Geometry check sheet. Reference: the model listing, model coordinates, mm. A direction names the side the tool comes from. Round coordinates to 2 decimals unless told otherwise and drop trailing zeros. Write each loop counter-clockwise with the first axis right and the second up, starting at its lowest first coordinate (ties: lowest second). Pieces come first, ordered by that corner, then holes. Notation, with made-up numbers: M 19.5,-33 L 27.5,-33 A18 ccw 27.5,-22 Z; hole C -7.5,8.25 d11. An arc over 180 degrees is marked long. Put each result on its own line as item: value. Start each with the question number.
(1) Tool access check on faces 4 (the flat face through (-40, 0, 13)), 5 (the flat face through (15, -15, 37)), 6 (the flat face through (40, 0, 13)). Record the directions out of +Z, -Z, +X, -X, +Y, -Y that give a thin tool (end or side, any length) a straight path to the whole face; none if there is none.
(2) Mould release check, pull along Y, two halves, no side actions. Record for faces 1 (the flat face through (50, -13, 13)), 2 (the flat face through (15, 15, 37)), 3 (the flat face through (-60, 21, 12)): pulls with the +Y half, pulls with the -Y half, needs draft (parallel to the pull), parting line crosses it, or undercut.
(3) Section check B-B on x = -50.5. Record the cut outline in (y, z), then the cut area to 3 significant figures.
(4) Section check D-D on x = 27. Record the cut outline in (y, z).
(5) Gauge pin test, flat ends, axial feed: pin 1 (10 mm diameter, centred on x = -30, y = -21.5, fed in from +Z); pin 2 (7.5 mm diameter, centred on y = 2, z = 14.5, fed in from +X); pin 3 (5 mm diameter, centred on x = -20.5, z = 28.5, fed in from -Y). Record the tip position at first contact, or that the pin passes through.
(6) Material ranges on probe 1 along Y at (x, z) = (-44.5, 9.5); probe 2 along Z at (x, y) = (-30.5, -11.5); probe 3 along X at (y, z) = (9, 15), recorded low to high.
(7) Section check A-A on z = 32.5. Record the cut outline in (x, y).
(8) Section check C-C on y = 22.5. Record the cut outline in (x, z).
from build123d import *

# Parameters (mm, degrees)
F0_W      = 120
F0_H      = 60
F1_DEPTH  = 25
F2_W      = 20
F2_H      = 26
F3_DEPTH  = 25.001
F4_W      = 20
F4_H      = 26
F5_DEPTH  = 25.001
F7_DEPTH  = 25
F8_DEPTH  = 35.001
F10_DEPTH = 25


with BuildPart() as f1:
    # F0 (on Top) → F1 (new body)
    with BuildSketch(Plane.XY):
        Rectangle(F0_W, F0_H)
    extrude(amount=F1_DEPTH)

    # F2 (on face) → F3 (cut, through all)
    with BuildSketch(Plane.XY.offset(25)):
        with Locations((50, 0)):
            Rectangle(F2_W, F2_H)
    extrude(amount=-F3_DEPTH, mode=Mode.SUBTRACT)

    # F4 (on face) → F5 (cut, through all)
    with BuildSketch(Plane.XY.offset(25)):
        with Locations((-50, 0)):
            Rectangle(F4_W, F4_H)
    extrude(amount=-F5_DEPTH, mode=Mode.SUBTRACT)

    # F6 (on face) → F7 (cut)
    with BuildSketch(Plane.XZ.offset(30)):
        with BuildLine():
            Line((-18, 0), (18, 0))
            ThreePointArc((18, 0), (0, 18), (-18, 0))
        make_face()
    extrude(amount=-F7_DEPTH, mode=Mode.SUBTRACT)

    # F8 (cut, through all): a face of the model
    f8_faces = [f1.faces().sort_by_distance(p)[0] for p in [
        (0, -5, 7.6394372684),
    ]]
    extrude(f8_faces, amount=-F8_DEPTH, mode=Mode.SUBTRACT)

    # F9 (on face) → F10 (join)
    with BuildSketch(Plane.XY.offset(25)):
        with BuildLine():
            ThreePointArc((0, 11), (7.7781745931, 7.7781745931), (11, 0))
            Line((11, 0), (30, 0))
            Line((30, 0), (0, 30))
            Line((0, 30), (0, 11))
        make_face()
        with BuildLine():
            ThreePointArc((-11, 0), (-7.7781745931, 7.7781745931), (0, 11))
            Line((0, 11), (0, 30))
            Line((0, 30), (-30, 0))
            Line((-30, 0), (-11, 0))
        make_face()
        with BuildLine():
            Line((0, -30), (0, -11))
            ThreePointArc((0, -11), (-7.7781745931, -7.7781745931), (-11, 0))
            Line((-11, 0), (-30, 0))
            Line((-30, 0), (0, -30))
        make_face()
        with BuildLine():
            Line((30, 0), (11, 0))
            ThreePointArc((11, 0), (7.7781745931, -7.7781745931), (0, -11))
            Line((0, -11), (0, -30))
            Line((0, -30), (30, 0))
        make_face()
    extrude(amount=F10_DEPTH)


solid = f1.part
Answers follow:
1. face 4: +Z, -Z, -X
1. face 5: +Z, +X, -Y
1. face 6: +Z, -Z, +X
2. face 1: undercut
2. face 2: pulls with the +Y half
2. face 3: needs draft
3. outline: M -30,0 L -13,0 L -13,25 L -30,25 Z; M 13,0 L 30,0 L 30,25 L 13,25 Z
3. area: 850 mm^2
4. outline: M -30,0 L 30,0 L 30,25 L 3,25 L 3,50 L -3,50 L -3,25 L -30,25 Z
5. pin 1: stops at z = 25
5. pin 2: stops at x = 40
5. pin 3: stops at y = -12
6. probe 1: y = -30 to -13, 13 to 30
6. probe 2: z = 0 to 25
6. probe 3: x = -40 to -9.95, 9.95 to 40
7. outline: M -30,0 L 0,-30 L 30,0 L 0,30 Z; hole C 0,0 d22
8. outline: M -60,0 L -18,0 A18 cw 18,0 L 60,0 L 60,25 L 7.5,25 L 7.5,50 L -7.5,50 L -7.5,25 L -60,25 Z
